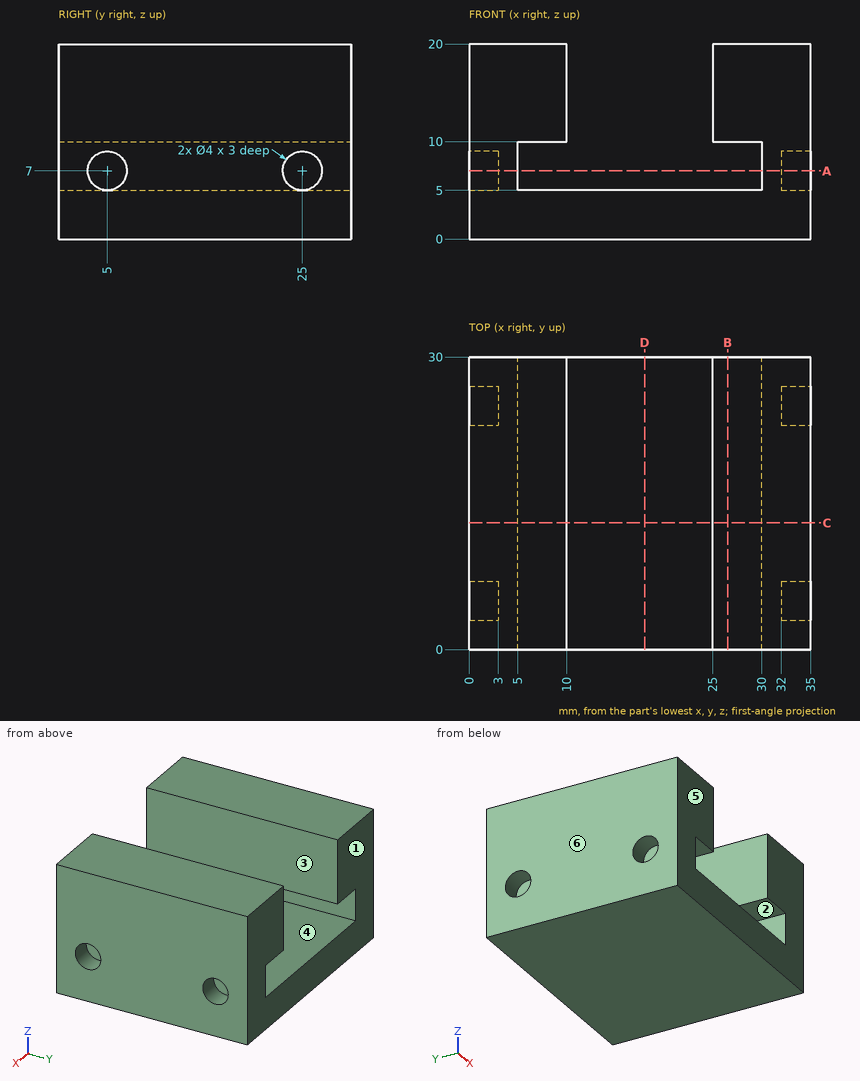
Geometry: see drawing. Coordinates: mm, zero at the bounding-box minimum. A direction names the side the tool comes from. Round coordinates to 2 decimals unless told otherwise and drop trailing zeros. Write each loop counter-clockwise with the first axis right and the second up, starting at its lowest first coordinate (ties: lowest second). Pieces come first, ordered by that corner, then holes. Notation, with made-up numbers: M 35,14.5 L 74,14.5 A20 ccw 74,31.5 Z; hole C -8,5.25 d5. An arc over 180 degrees is marked long. Answer as a JSON object with one key per item and string values. Group by question number.
(1) Section query A-A on z = 7. Output: boundary loops of the cut face in (x, y), then the cut area to 3 significant figures.
(2) Section query C-C on y = 13. Output: boundary loops of the cut face in (x, z), then the cut area to 3 significant figures.
(3) Ray query, line 1 (Y direction, x = 2.2, z = 7); line 2 (Z direction, x = 28.5, y = 19); line 3 (X direction, y = 16, z = 10.25). Return the intervals inside material, ascending. Write a range as [from, to].
(4) Mould query, pull axis X, two halves, no side actions, for the marked faces 4, 5 and 6. Classes: +X half, -X half, draft (parallel to the pull), parting line (faces both ways), or undercut.
(5) Reachability of the marked faces 1, 2 and 3 from +Z, -Z, +X, -X, +Y, -Y: full face, straight path, thin tool, end or side. Return the list, or none.
(6) First-contact query: pin 1 (1.2 mm diameter, centred on y = 24.5, z = 6.5, fed in from -X); pin 2 (3 mm diameter, centred on x = 12.5, z = 12, fed in from +Y); pin 3 (1 mm diameter, centred on y = 25.5, z = 7, fed in from +X). Flat tips, straight axial feed; report the tip coordinate or a pass-through.
(7) Section query B-B on x = 26.5. Output: boundary loops of the cut face in (y, z).
(8) Section query D-D on x = 18. Output: boundary loops of the cut face in (y, z).
Computed values:
{
 "1": {"outline": "M 0,0 L 5,0 L 5,30 L 0,30 L 0,27 L 3,27 L 3,23 L 0,23 L 0,7 L 3,7 L 3,3 L 0,3 Z; M 30,0 L 35,0 L 35,3 L 32,3 L 32,7 L 35,7 L 35,23 L 32,23 L 32,27 L 35,27 L 35,30 L 30,30 Z", "area": "252 mm^2"},
 "2": {"outline": "M 0,0 L 35,0 L 35,20 L 25,20 L 25,10 L 30,10 L 30,5 L 5,5 L 5,10 L 10,10 L 10,20 L 0,20 Z", "area": "425 mm^2"},
 "3": {"line 1": "[0, 3], [7, 23], [27, 30]", "line 2": "[0, 5], [10, 20]", "line 3": "[0, 10], [25, 35]"},
 "4": {"face 4": "undercut", "face 5": "draft", "face 6": "-X half"},
 "5": {"face 1": "+Z, -Z, +X, -X, +Y", "face 2": "+Y, -Y", "face 3": "+Z, +Y, -Y"},
 "6": {"pin 1": "x = 3", "pin 2": "through", "pin 3": "x = 32"},
 "7": {"outline": "M 0,0 L 30,0 L 30,5 L 0,5 Z; M 0,10 L 30,10 L 30,20 L 0,20 Z"},
 "8": {"outline": "M 0,0 L 30,0 L 30,5 L 0,5 Z"}
}
